Design review of the part built by this model. Coordinates are the model's own, in mm. A direction names the side the tool comes from. Give positions to 0.01 mm unless a question says otherwise; leave off trailing zeros. Loops run counter-clockwise (first coordinate to the right, second up) from the corner with the lowest first, then second, coordinate; pieces in that order, holes last. Notation, with made-up numbers: M 79.5,46 L 108.5,46 A15 cw 108.5,53 Z; hole C 67.25,83 d9. An arc over 180 degrees is marked long. Use a Markdown table: item, result. Add a question column.
(1) Insertion check: pin 1 Ø10 at (x, z) = (7, 31.5) entering from -Y; pin 2 Ø9.5 at (y, z) = (2, 50) entering from -X; pin 3 Ø17 at (y, z) = (0, 46) entering from +X; pin 4 Ø1 at (x, y) = (16.5, -12.5) entering from -Z. Each pin has a flat end and moves straight along its axis. Give the tip position at first contact, or say it passes through.
(2) Add section A-A, the plane z = 46. Give the boundary of the cut face in (x, y), then the cut area to 3 significant figures.
(3) For probe 1 along X at (y, z) = (9.5, 36); probe 2 along Y at (x, z) = (26.25, 46); probe 3 along X at (y, z) = (13.5, 6), list the stretches that pass through material, from the lowest coordinate up.
(4) For faces 5 (the face through (-31.5, 0, 38)), 6 (the face through (44, 7, 13)), 7 (the face through (33, 0, 0)), 8 (the face through (-17.5, 0, 8)), 9 (the face through (17.5, 0, 39)), list the 3-axis set-ups (+Z, -Z, +X, -X, +Y, -Y) from which the entire face can be reached by the end or side of a thin tool; tool diameter is ignored.
(5) Add section B-B, the plane y = -5. State how many separate pieces and enclosed holes the cut face has, then the cut area to 3 significant figures.
(6) Draft analysis for pull direction Y (two halves, no side actions). For faces 1 (the face through (-56.5, 6, 7)), 2 (the face through (37, 0, 7)), 3 (the face through (1, 16, 20)), 4 (the face through (-50, 0, 7)), state which applies: pulls with the +Y half, pulls with the -Y half, needs draft (parallel to the pull), parting line crosses it, or undercut.
(7) Add section C-C, the plane z = 35.5. Give the boundary of the cut face in (x, y).
(8) Add section D-D, the plane x = 25. Give the boundary of the cut face in (y, z), then the cut area to 3 significant figures.
```python
from build123d import *

# Parameters (mm, degrees)
F0_R     = 6.5
F1_DEPTH = 56.5
F2_W     = 25
F2_H     = 51
F2_W_2   = 35
F2_H_2   = 17
F2_H_3   = 34
F3_DEPTH = 32.001
F4_R     = 6.5
F5_DEPTH = 13.001
F6_R     = 6.5
F7_DEPTH = 13.001


with BuildPart() as f1:
    # F0 (on Right) → F1 (new body, symmetric)
    with BuildSketch(Plane.YZ):
        with BuildLine():
            Line((-16, 0), (16, 0))
            Line((16, 0), (16, 53.588723))
            ThreePointArc((16, 53.588723), (9.544562, 61.168038), (0, 64))
            ThreePointArc((0, 64), (-9.544562, 61.168038), (-16, 53.588723))
            Line((-16, 53.588723), (-16, 0))
        make_face()
        with Locations((0, 46)):
            Circle(F0_R, mode=Mode.SUBTRACT)
    extrude(amount=F1_DEPTH, both=True)

    # F2 (on face) → F3 (cut, through all)
    with BuildSketch(Plane(origin=(0, 16, 0), x_dir=(-1, 0, 0), z_dir=(0, 1, 0))):
        with Locations((44, 38.5)):
            Rectangle(F2_W, F2_H)
        with Locations((-44, 38.5)):
            Rectangle(F2_W, F2_H)
        with Locations((0, 8.5)):
            Rectangle(F2_W_2, F2_H_2)
        with Locations((0, 47)):
            Rectangle(F2_W_2, F2_H_3)
    extrude(amount=-F3_DEPTH, mode=Mode.SUBTRACT)

    # F4 (on face) → F5 (cut, through all)
    with BuildSketch(Plane.XY.offset(13)):
        with Locations((-43.5, 0)):
            Circle(F4_R)
        Polygon((-56.5, -3), (-56.5, -16), (-43.5, -16), align=None)
    extrude(amount=-F5_DEPTH, mode=Mode.SUBTRACT)

    # F6 (on face) → F7 (cut, through all)
    with BuildSketch(Plane.XY.offset(13)):
        with Locations((43.5, 0)):
            Circle(F6_R)
        Polygon((56.5, -3), (43.5, -16), (56.5, -16), align=None)
    extrude(amount=-F7_DEPTH, mode=Mode.SUBTRACT)


solid = f1.part
```
Established:
| question | item | result |
|---|---|---|
| 1 | pin 1 | y = -16 |
| 1 | pin 2 | x = -31.5 |
| 1 | pin 3 | x = 31.5 |
| 1 | pin 4 | z = 17 |
| 2 | outline | M -31.5,-16 L -17.5,-16 L -17.5,-6.5 L -31.5,-6.5 Z; M -31.5,6.5 L -17.5,6.5 L -17.5,16 L -31.5,16 Z; M 17.5,-16 L 31.5,-16 L 31.5,-6.5 L 17.5,-6.5 Z; M 17.5,6.5 L 31.5,6.5 L 31.5,16 L 17.5,16 Z |
| 2 | area | 532 mm^2 |
| 3 | probe 1 | -31.5 to -17.5, 17.5 to 31.5 |
| 3 | probe 2 | -16 to -6.5, 6.5 to 16 |
| 3 | probe 3 | -56.5 to -17.5, 17.5 to 56.5 |
| 4 | face 5 | +Z, -X, +Y, -Y |
| 4 | face 6 | +Z, +X, +Y, -Y |
| 4 | face 7 | -Z, +X, -X, +Y, -Y |
| 4 | face 8 | -Z, +Y, -Y |
| 4 | face 9 | +Z, +Y, -Y |
| 5 | separate pieces | 5 |
| 5 | enclosed holes | 0 |
| 5 | area | 2,380 mm^2 |
| 6 | face 1 | needs draft |
| 6 | face 2 | undercut |
| 6 | face 3 | pulls with the +Y half |
| 6 | face 4 | undercut |
| 7 | outline | M -31.5,-16 L -17.5,-16 L -17.5,16 L -31.5,16 Z; M 17.5,-16 L 31.5,-16 L 31.5,16 L 17.5,16 Z |
| 8 | outline | M -16,0 L 16,0 L 16,53.59 A17.5 ccw -16,53.59 Z; hole C 0,46 d13 |
| 8 | area | 1,820 mm^2 |
